Build history of the part. All positions in model axes, mm. Face numbers are marked on the shaded views. Round coordinates to 2 decimals unless told otherwise and drop trailing zeros. Write each loop counter-clockwise with the first axis right and the second up, starting at its lowest first coordinate (ties: lowest second). Pieces come first, ordered by that corner, then holes.
from build123d import *

# Parameters (mm, degrees)
EXTRUDE_1_DEPTH = 1.2
SKETCH_3_R      = 0.5
EXTRUDE_2_DEPTH = 5.8
CHAMFER_1_SIZE  = 0.2


with BuildPart() as part:
    # Эскиз1 → Повернуть1 (revolve)
    with BuildSketch(Plane(origin=(0, 0, 0), x_dir=(0, 0, -1), z_dir=(1, 0, 0))):
        with BuildLine():
            Line((0, 1.2), (-7.05, 1.2))
            Line((-7.05, 1.2), (-7.25, 1.4))
            Line((-7.25, 1.4), (-7.65, 1))
            Line((-7.65, 1), (-8.65, 1))
            ThreePointArc((-8.65, 1), (-8.561771126, 4.984856949), (-8.297257426, 8.96190381))
            ThreePointArc((-8.297257426, 8.96190381), (-8.072581915, 9.416397457), (-7.6, 9.6))
            Line((-7.6, 9.6), (-5.1, 9.6))
            Line((-5.1, 9.6), (-5.1, 8.7))
            Line((-5.1, 8.7), (0, 8.7))
            Line((0, 8.7), (0, 1.2))
        make_face()
    revolve(axis=Axis((0, 8.7, 0), (0, -1, 0)))

    # Эскиз2 → Бобышка-Вытянуть1 (add)
    with BuildSketch(Plane.XZ.offset(-1.2)):
        with BuildLine():
            ThreePointArc((-2.368807717, 2.368807717), (-2.368807717, 4.384062043), (-4.384062043, 4.384062043))
            ThreePointArc((-4.384062043, 4.384062043), (-6.2, 0), (-4.384062043, -4.384062043))
            ThreePointArc((-4.384062043, -4.384062043), (-2.368807717, -4.384062043), (-2.368807717, -2.368807717))
            ThreePointArc((-2.368807717, -2.368807717), (-3.35, 0), (-2.368807717, 2.368807717))
        make_face()
        with BuildLine():
            ThreePointArc((4.384062043, -4.384062043), (5.728053102, -2.372637281), (6.2, 0))
            ThreePointArc((6.2, 0), (5.728053102, 2.372637281), (4.384062043, 4.384062043))
            ThreePointArc((4.384062043, 4.384062043), (2.368807717, 4.384062043), (2.368807717, 2.368807717))
            ThreePointArc((2.368807717, 2.368807717), (3.094996434, 1.281989498), (3.35, 0))
            ThreePointArc((3.35, 0), (3.094996434, -1.281989498), (2.368807717, -2.368807717))
            ThreePointArc((2.368807717, -2.368807717), (2.368807717, -4.384062043), (4.384062043, -4.384062043))
        make_face()
    extrude(amount=EXTRUDE_1_DEPTH)

    # Эскиз3 → Бобышка-Вытянуть2 (add)
    with BuildSketch(Plane.XZ):
        with Locations(Location((-4.75, 0, 0), (0, 0, 270))):
            Circle(SKETCH_3_R)
        with Locations(Location((-3.358757211, 3.358757211, 0), (0, 0, 270))):
            Circle(SKETCH_3_R)
        with Locations(Location((-3.358757211, -3.358757211, 0), (0, 0, 270))):
            Circle(SKETCH_3_R)
        with Locations(Location((3.358757211, 3.358757211, 0), (0, 0, 90))):
            Circle(SKETCH_3_R)
        with Locations(Location((4.75, 0, 0), (0, 0, 90))):
            Circle(SKETCH_3_R)
        with Locations(Location((3.358757211, -3.358757211, 0), (0, 0, 90))):
            Circle(SKETCH_3_R)
    extrude(amount=EXTRUDE_2_DEPTH)

    # Фаска1
    chamfer_1_edges = [part.edges().sort_by_distance(p)[0] for p in [
        (-4.75, -5.8, 0.5),
        (-3.358757211, -5.8, 3.858757211),
        (-3.358757211, -5.8, -2.858757211),
        (3.358757211, -5.8, 2.858757211),
        (4.75, -5.8, -0.5),
        (3.358757211, -5.8, -3.858757211),
    ]]
    chamfer(chamfer_1_edges, length=CHAMFER_1_SIZE)


solid = part.part
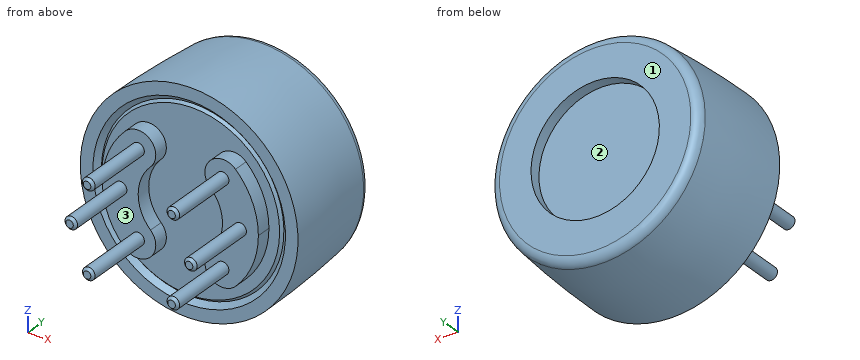
1) Pin check, flat tips, straight feed: pin 1 Ø1.3 at (x, z) = (-3.5, 0.5) entering from -Y; pin 2 Ø1 at (y, z) = (4, -0.5) entering from +X; pin 3 Ø5 at (x, z) = (2.5, -0.5) entering from +Y. Stop position of each tip, or through.
Results:
pin 1: stops at y = 0
pin 2: stops at x = 8.61
pin 3: stops at y = 8.7
2) Wall check: L1, parallel to Z at x = 0, y = 9; L2, parallel to Y at x = 0.5, z = -2.5; L3, parallel to Z at x = 3, y = -2. Give the ranges that are in metal, low to high.
Results:
L1: z = -8.29 to -5.1, 5.1 to 8.29
L2: y = 1.2 to 8.7
L3: z = -3.71 to -3.01, 3.01 to 3.71
3) Mould opens along Z. For the marked faces 1, 2 and 3 say: released by +Z, released by -Z, zero draft, split by the parting line, or undercut.
Results:
face 1: zero draft
face 2: undercut
face 3: undercut
4) Slice it at A-A (y = -4.75). Write the cut outline in (x, z), plus the area to 3 significant figures.
Results:
outline: circle Ø1 at (-4.75, 0); circle Ø1 at (-3.36, -3.36); circle Ø1 at (-3.36, 3.36); circle Ø1 at (3.36, -3.36); circle Ø1 at (3.36, 3.36); circle Ø1 at (4.75, 0)
area: 4.71 mm2
